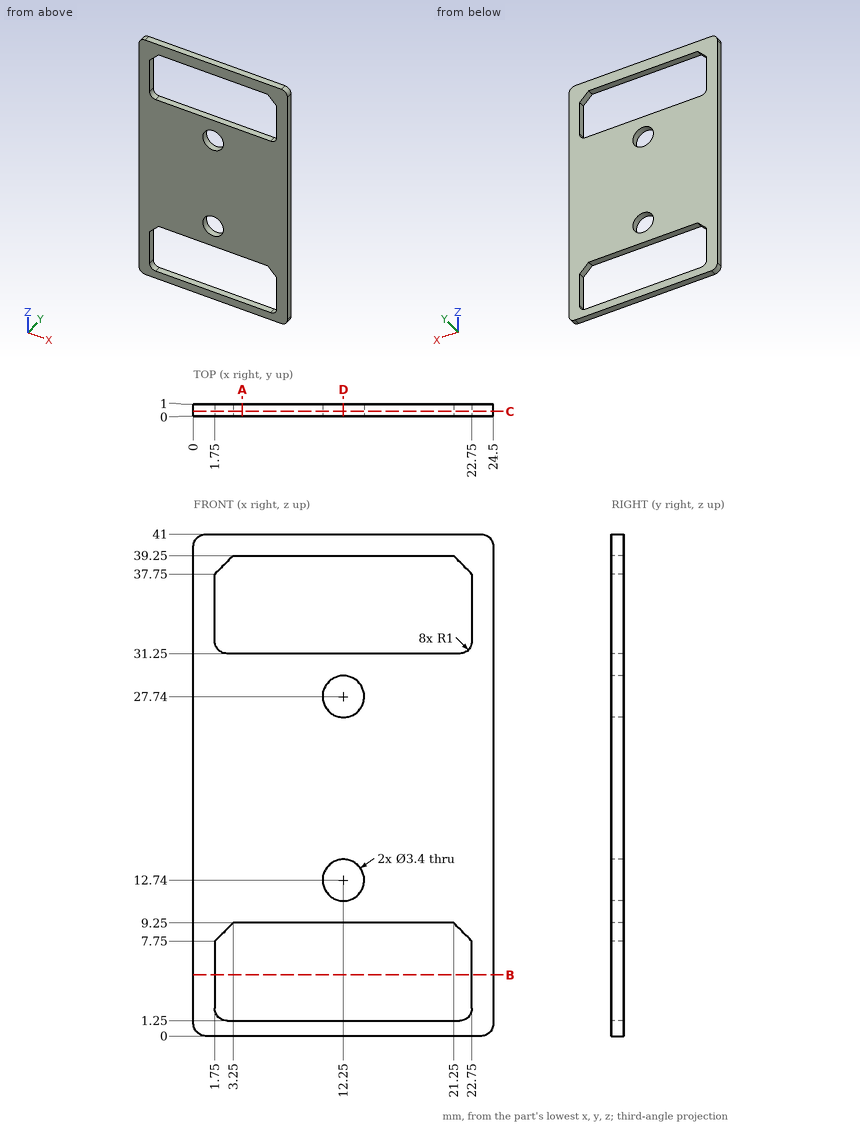
Part print with two shaded views. Sizes in mm from the minimum x, y, z corner. Round coordinates to 2 decimals unless told otherwise and drop trailing zeros. Order: outer loops, then holes, each group sorted by start corner. A loop starts at its lowest first (then second) coordinate and runs counter-clockwise, first axis right, second up. Notation, with made-up numbers: (88, 28) -> (128, 28) arc R20 cw to (128, 48) -> close; hole circle Ø7 at (61, 61). An arc over 180 degrees is marked (long way). One line per question, with ' | ' between items.
Q1. Slice it at D-D (x = 12.25). Write the cut outline in (y, z), then the cut area to 3 significant figures.
Completed:
outline: (0, 0) -> (1, 0) -> (1, 1.25) -> (0, 1.25) -> close; (0, 9.25) -> (1, 9.25) -> (1, 11.04) -> (0, 11.04) -> close; (0, 14.44) -> (1, 14.44) -> (1, 26.04) -> (0, 26.04) -> close; (0, 29.44) -> (1, 29.44) -> (1, 31.25) -> (0, 31.25) -> close; (0, 39.25) -> (1, 39.25) -> (1, 41) -> (0, 41) -> close | area: 18.2 mm^2
Q2. Slice it at A-A (x = 4). Write the cut outline in (y, z), then the cut area to 3 significant figures.
Completed:
outline: (0, 0) -> (1, 0) -> (1, 1.25) -> (0, 1.25) -> close; (0, 9.25) -> (1, 9.25) -> (1, 31.25) -> (0, 31.25) -> close; (0, 39.25) -> (1, 39.25) -> (1, 41) -> (0, 41) -> close | area: 25.0 mm^2
Q3. Drop a flat-ended pin along its axis: pin 1 (2 mm diameter, centred on x = 12.25, z = 27.74, fed in from +Y). Give the stop position or say it passes through.
Completed:
pin 1: passes through
Q4. Slice it at C-C (y = 0.4). Write the cut outline in (x, z).
Completed:
outline: (0, 1) arc R1 ccw to (1, 0) -> (23.5, 0) arc R1 ccw to (24.5, 1) -> (24.5, 40) arc R1 ccw to (23.5, 41) -> (1, 41) arc R1 ccw to (0, 40) -> close; hole (1.75, 2.25) arc R1 ccw to (2.75, 1.25) -> (21.75, 1.25) arc R1 ccw to (22.75, 2.25) -> (22.75, 7.75) -> (21.25, 9.25) -> (3.25, 9.25) -> (1.75, 7.75) -> close; hole (1.75, 32.25) arc R1 ccw to (2.75, 31.25) -> (21.75, 31.25) arc R1 ccw to (22.75, 32.25) -> (22.75, 37.75) -> (21.25, 39.25) -> (3.25, 39.25) -> (1.75, 37.75) -> close; hole circle Ø3.4 at (12.25, 12.74); hole circle Ø3.4 at (12.25, 27.74)
Q5. Slice it at B-B (z = 5). Write the cut outline in (x, y).
Completed:
outline: (0, 0) -> (1.75, 0) -> (1.75, 1) -> (0, 1) -> close; (22.75, 0) -> (24.5, 0) -> (24.5, 1) -> (22.75, 1) -> close
Q6. Probe probe 1 along Z at (x, y) = (4.5, 0.45); probe 2 along Z at (x, y) = (12.25, 0.35); probe 3 along X at (y, z) = (0.8, 7). List the from-to ranges inside material, lowest first.
Completed:
probe 1: z = 0 to 1.25, 9.25 to 31.25, 39.25 to 41 | probe 2: z = 0 to 1.25, 9.25 to 11.04, 14.44 to 26.04, 29.44 to 31.25, 39.25 to 41 | probe 3: x = 0 to 1.75, 22.75 to 24.5
